Work out the finished part from the listing and answer in its coordinate system (mm). A direction names the side the tool comes from. Give positions to 0.01 mm unless a question says otherwise; leave off trailing zeros. Write each loop counter-clockwise with the first axis right and the second up, starting at its lowest first coordinate (ties: lowest second). Pieces come first, ordered by that corner, then holes. Notation, with made-up numbers: (-27.5, 42.5) - (7.5, 42.5) arc R15 ccw to (7.5, 46.5) - close; hole circle Ø1 at (-35, 43.25). An arc over 180 degrees is marked (long way). Write item = value, one per line.
from build123d import *

# Parameters (mm, degrees)
ESQUISSE1_R             = 12.2
BOSS_EXTRU_1_DEPTH      = 26.9
ESQUISSE2_R             = 3.5
BOSS_EXTRU_2_DEPTH      = 2.5
ESQUISSE3_R             = 2
BOSS_EXTRU_3_DEPTH      = 10
ENL_V_MAT_EXTRU_1_DEPTH = 8


with BuildPart() as part:
    # Esquisse1 → Boss.-Extru.1 (new body, symmetric)
    with BuildSketch(Plane.XY):
        Circle(ESQUISSE1_R)
    extrude(amount=BOSS_EXTRU_1_DEPTH, both=True)

    # Esquisse2 → Boss.-Extru.2 (add)
    with BuildSketch(Plane.XY.offset(26.9)):
        Circle(ESQUISSE2_R)
    extrude(amount=BOSS_EXTRU_2_DEPTH)

    # Esquisse3 → Boss.-Extru.3 (add)
    with BuildSketch(Plane.XY.offset(29.4)):
        Circle(ESQUISSE3_R)
    extrude(amount=BOSS_EXTRU_3_DEPTH)

    # Esquisse4 → Enlèv. mat.-Extru.1 (cut)
    with BuildSketch(Plane.XY.offset(39.4)):
        with BuildLine():
            Line((-1.233818862, -1.574068301), (1.407495119, -1.42090024))
            ThreePointArc((1.407495119, -1.42090024), (0.115784171, -1.996645694), (-1.233818862, -1.574068301))
        make_face()
    extrude(amount=-ENL_V_MAT_EXTRU_1_DEPTH, mode=Mode.SUBTRACT)


solid = part.part
1. Straight lines are drawn through the part: line 1 (Z direction, x = -1.75, y = -2.25); line 2 (Z direction, x = 4.75, y = 4.75); line 3 (Y direction, x = 4.75, z = 24). For each, find the intervals that lie inside material, in ascending order.
Solution:
line_1 = -26.9 to 29.4
line_2 = -26.9 to 26.9
line_3 = -11.24 to 11.24
2. Find section D-D, the plane x = -4.5. Give the vertices of the cut face in (y, z).
Solution:
outline = (-11.34, -26.9) - (11.34, -26.9) - (11.34, 26.9) - (-11.34, 26.9) - close
3. Find section B-B, the plane x = 0. Give the vertices of the cut face in (y, z).
Solution:
outline = (-12.2, -26.9) - (12.2, -26.9) - (12.2, 26.9) - (3.5, 26.9) - (3.5, 29.4) - (2, 29.4) - (2, 39.4) - (-1.5, 39.4) - (-1.5, 31.4) - (-2, 31.4) - (-2, 29.4) - (-3.5, 29.4) - (-3.5, 26.9) - (-12.2, 26.9) - close
4. A tool of negligible diameter and unlimited length cuts with its end or side. For faces 1 (the flat face through (0.07, -1.5, 35.46)), 2 (the flat face through (0, 0, 39.4)), 3 (the cylindrical face through (3.233, -1.341, 28.132)), from which of +Z, -Z, +X, -X, +Y, -Y can it reach the whole face along a straight path? Write none if from no direction.
Solution:
face_1 = +Z, +X, -Y
face_2 = +Z, +X, -X, +Y, -Y
face_3 = +Z
5. Find section C-C, the plane z = -11. Give the vertices of the cut face in (x, y), then the cut area to 3 significant figures.
Solution:
outline = circle Ø24.4 at (0, 0)
area = 468 mm^2
6. Find section A-A, the plane y = 0. Give the vertices of the cut face in (x, z), then the cut area to 3 significant figures.
Solution:
outline = (-12.2, -26.9) - (12.2, -26.9) - (12.2, 26.9) - (3.5, 26.9) - (3.5, 29.4) - (2, 29.4) - (2, 39.4) - (-2, 39.4) - (-2, 29.4) - (-3.5, 29.4) - (-3.5, 26.9) - (-12.2, 26.9) - close
area = 1,370 mm^2
7. Given pin 1 (1.5 mm diameter, centred on y = -5.5, z = 15.5, fed in from -X); pin 2 (1.5 mm diameter, centred on x = 9.5, z = 18.5, fed in from +Y); pin 3 (10 mm diameter, centred on y = -6.5, z = 23, fed in from +X), each flat-ended and moving along its own axis, determine where each tip first touches the part or whether it passes through.
Solution:
pin_1 = -11.24
pin_2 = 8.5
pin_3 = 12.11
